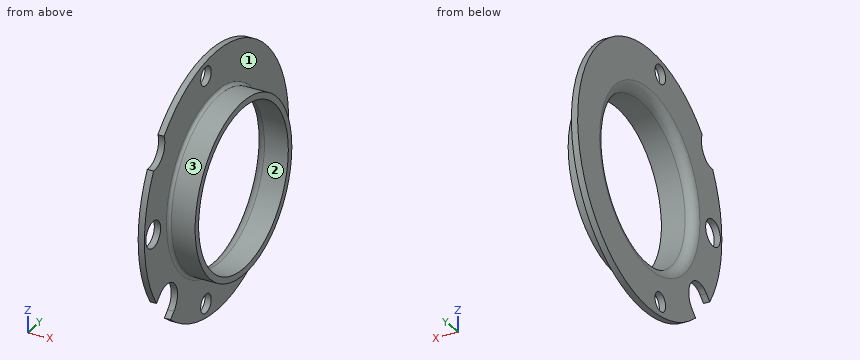
Autodesk Inventor part; units mm, degrees
ref_plane "YZ Plane" through (0, 0, 0) normal (1, 0, 0) x (0, 1, 0)
ref_plane "XZ Plane" through (0, 0, 0) normal (0, 1, 0) x (-1, 0, 0)
ref_plane "XY Plane" through (0, 0, 0) normal (0, 0, 1) x (1, 0, 0)
sketch "Sketch1" plane through (0, 0, 0) normal (0, 0, 1) x (1, 0, 0)
  line L0 (0, 20.5) -> (1, 20.5)
  line L1 (1, 20.5) -> (1, 12.75)
  line L2 (1, 12.75) -> (0, 12.75)
  line L3 (0, 12.75) -> (0, 20.5)
  line L4 (1, 12.75) -> (5.3, 12.75)
  line L5 (5.3, 12.75) -> (5.3, 13.75)
  line L6 (5.3, 13.75) -> (1, 13.75)
  line L7 (1, 13.75) -> (1, 12.75)
  line L8 (0, 0) -> (7.1603, 0)
  dimension "d0" = 41
  dimension "d2" = 27.5
  dimension "d3" = 1
  dimension "d4" = 5.3
revolve "Revolution1" add sketch "Sketch1" angle 360 about axis through (0, 0, 0) along (1, 0, 0)
fillet "Fillet1" radius 1.5 1 edges at (0, -12.75, 0)
fillet "Fillet1" radius 0.5 1 edges at (1, -13.75, 0)
sketch "Sketch2" plane through (0, 0, 0) normal (-1, 0, 0) x (0, 0, 1)
  line L0 (-18, -3) -> (18, -3) construction
  point P0 (0, 0)
  point P1 (0, -3)
  dimension "d8" = 36
  dimension "d9" = 3
hole "Hole1" at (0, -3, 18) at (0, -3, -18) direction (1, 0, 0) diameter 3 end through all
sketch "Sketch3" plane through (0, 0, 0) normal (-1, 0, 0) x (0, 0, 1)
  circle A0 centre (13, -17.7) radius 3
  circle A1 centre (-12.7, -14.1) radius 3
  line L0 (0, 0) -> (-12.7, -14.1) construction
  line L1 (-10.4709, -16.1078) -> (-11.3429, -17.0759)
  circle A2 centre (0, 0) radius 20.5
  line L2 (-14.9291, -12.0922) -> (-15.8011, -13.0604)
  dimension "d17" = 13
  dimension "d18" = 17.7
  dimension "d19" = 12.7
  dimension "d20" = 14.1
  dimension "d21" = 6
  dimension "d22" = 6
extrude "Extrusion1" cut sketch "Sketch3" against normal through all contours A0 A2 | A2 A0 | A2 A1 L1 | L2 A1 A2 | A1 A2 | A1 A2
sketch "Sketch4" plane through (0, 0, 0) normal (1, 0, 0) x (0, 1, 0)
  line L0 (0, 0) -> (-18, 0) construction
  dimension "d25" = 18
hole "Hole2" at (0, -18, 0) direction (1, 0, 0) diameter 4.2 end through all
properties part number "403-02" material "Aluminum-6061"
Part model, mm, in its own coordinate system. Face numbers are marked on the shaded views. Round coordinates to 2 decimals unless told otherwise and drop trailing zeros. Order: outer loops, then holes, each group sorted by start corner. A loop starts at its lowest first (then second) coordinate and runs counter-clockwise, first axis right, second up. Notation, with made-up numbers: M -19.5,88.5 L 27.5,88.5 A18 ccw 27.5,103.5 Z; hole C 60,85.5 d2. An arc over 180 degrees is marked long. Put each result on its own line as item: value. Start each with the question number.
1. Slice it at B-B on x = 3.05. List the corners of the cut face in (y, z), then the cut area to 3 significant figures.
2. Slice it at C-C on z = -17. List the corners of the cut face in (x, y), then the cut area to 3 significant figures.
3. Drop a flat-ended pin along its axis: pin 1 (3 mm diameter, centred on y = 1.5, z = 10, fed in from +X). Give the stop position or say it passes through.
4. Drill centre lines: probe 1 along Z at (x, y) = (0.4, -3); probe 2 along Z at (x, y) = (0.65, -3); probe 3 along Y at (x, z) = (0.6, 0). Where is each one in solid material? Low to high. Write a range as [from, to].
5. Slice it at A-A on z = 18. List the corners of the cut face in (x, y).
6. Two-plate mould, pull along Z, no slides. Class the marked faces 1, 2 and 3: +Z half, -Z half, draft (parallel to the pull), parting line (faces both ways), or undercut.
7. Slice it at D-D on y = -3. State how many separate pieces and enclosed holes the cut face has, then the cut area to 3 significant figures.
Findings:
1. outline: C 0,0 d27.5; hole C 0,0 d25.5
1. area: 83.3 mm2
2. outline: M 0,-11.46 L 1,-11.46 L 1,-4.12 L 0,-4.12 Z; M 0,-1.88 L 1,-1.88 L 1,11.46 L 0,11.46 Z
2. area: 20.7 mm2
3. pin 1: through
4. probe 1: [-20.28, -19.5], [-16.5, -12.89], [12.89, 16.5], [19.5, 20.28]
4. probe 2: [-20.28, -19.5], [-16.5, -12.66], [12.66, 16.5], [19.5, 20.28]
4. probe 3: [-20.5, -20.1], [-15.9, -13.05], [13.05, 20.5]
5. outline: M 0,-9.81 L 1,-9.81 L 1,-4.5 L 0,-4.5 Z; M 0,-1.5 L 1,-1.5 L 1,9.81 L 0,9.81 Z
6. face 1: draft
6. face 2: undercut
6. face 3: parting line
7. separate pieces: 4
7. enclosed holes: 0
7. area: 17.7 mm2
